Answer from the drawing. Dimensions are ordinates in mm from the lowest x, y and z of the part. Coordinates: 2 decimals unless noted, no trailing zeros. Write each loop counter-clockwise with the first axis right and the second up, starting at its lowest first coordinate (ties: lowest second). Pieces come first, ordered by that corner, then holes.
(1) Straight lines are drawn through the part: line 1 (X direction, y = 5.25, z = 55); line 2 (Y direction, x = 19, z = 15); line 3 (Z direction, x = 19.5, y = 1.5). For each, find the intervals that lie inside material, in ascending order.
(2) The part is cut by section A-A on x = 28.8. Determine the outline of the cut face in (y, z), plus the area to 3 significant figures.
(3) The part is cut by section B-B on z = 44. Determine the outline of the cut face in (x, y), plus the area to 3 significant figures.
(4) For a pull along Z with two mould halves and no side action, classify the marked faces 1 and 2 as +Z half, -Z half, draft (parallel to the pull), parting line (faces both ways), or undercut.
(5) Given P1, Ø16.5, axis at x = 26, z = 43, coming from the -Y side; P2, Ø1.5, axis at x = 38, y = 3.5, coming from the -Z side; P3, Ø4, axis at x = 35, y = 7, coming from the -Z side, each flat-ended and moving along its own axis, determine where each tip first touches the part or whether it passes through.
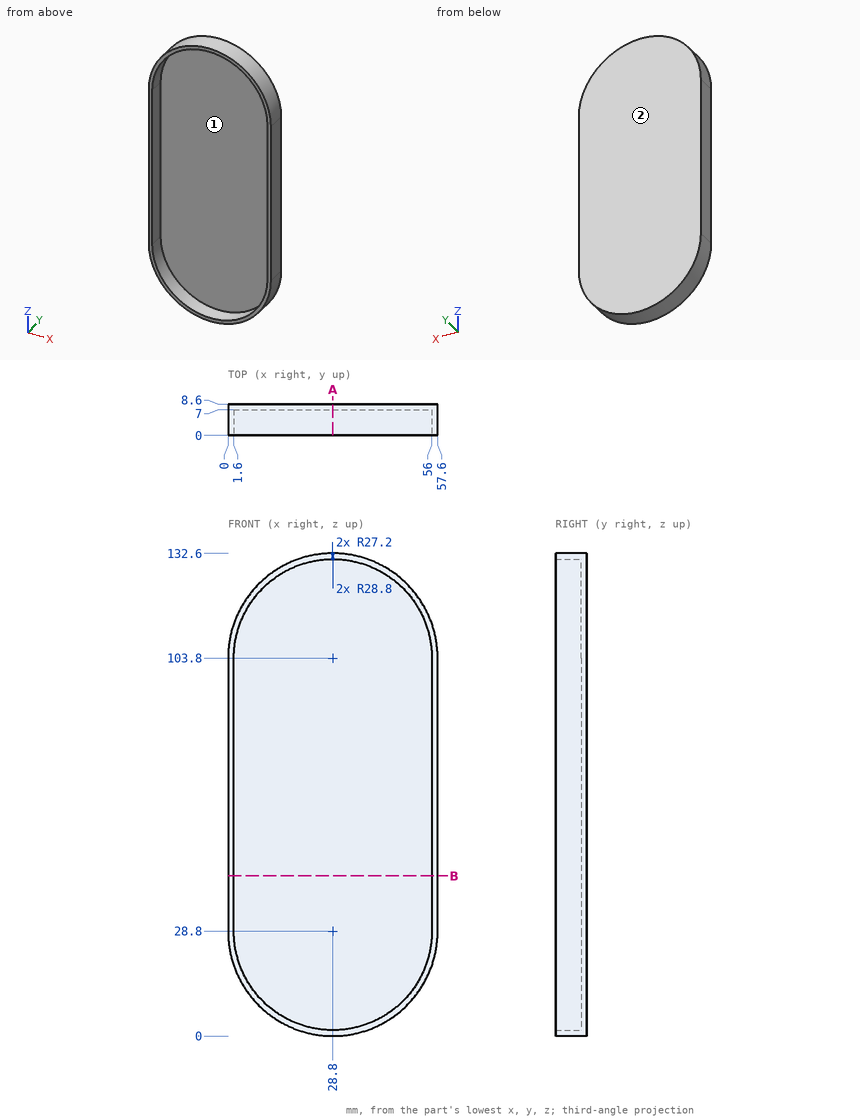
Model answer:
1. line 1: x = 0 to 1.6, 56 to 57.6
1. line 2: y = 7 to 8.6
1. line 3: z = 1.54 to 3.24, 129.36 to 131.06
2. outline: (0, 0) - (8.6, 0) - (8.6, 132.6) - (0, 132.6) - (0, 131) - (7, 131) - (7, 1.6) - (0, 1.6) - close
2. area: 235 mm2
3. outline: (0, 0) - (1.6, 0) - (1.6, 7) - (56, 7) - (56, 0) - (57.6, 0) - (57.6, 8.6) - (0, 8.6) - close
3. area: 115 mm2
4. face 1: undercut
4. face 2: draft
5. P1: stops at y = 7
5. P2: stops at z = 1.27
5. P3: stops at z = 0.31
